Can you work these out from the model? Positions are in its coordinate system, mm. Face numbers are marked on the shaded views. A direction names the side the tool comes from. Round coordinates to 2 decimals unless told otherwise and drop trailing zeros. Order: outer loops, then holes, each group sorted by start corner. A loop starts at its lowest first (then second) coordinate and runs counter-clockwise, first axis right, second up. Notation, with made-up numbers: (6.25, 24.5) -> (43.25, 24.5) arc R19 ccw to (43.25, 30.5) -> close; hole circle Ø2 at (57, 17). An arc over 180 degrees is marked (long way). Use a Markdown table: item, result. Add a question column.
Q1. If we section it at A-A on x = 3.5: List the corners of the cut face in (y, z) for me.
Q2. I need wall thicknesses on line 1 along Z through (x, y) = (-6.5, 7.25); line 2 along Z through (x, y) = (-3, 15); line 3 along X through (y, z) = (7.25, 32). Which ranges of each line are inside material? Lowest first, please. Write a range as [from, to].
Q3. I'm going to push flat-ended pins straight in: pin 1 Ø2 at (y, z) = (14.5, 20.5) entering from +X; pin 2 Ø4 at (y, z) = (7.5, 8.5) entering from -X; pin 3 Ø1 at (x, y) = (-12, 7.5) entering from -Z. Where does each tip first touch, or does it pass through?
Q4. If we section it at C-C on z = 52.5: List the corners of the cut face in (x, y) for me.
Q5. If we section it at D-D on y = 3: List the corners of the cut face in (x, z) for me.
Q6. If we section it at B-B on y = 8.75: List the corners of the cut face in (x, z) for me.
Q7. We'd pull the mould along X, two halves only. Please class the marked faces 1, 2 and 3: +X half, -X half, draft (parallel to the pull), parting line (faces both ways), or undercut.
Q8. For the marked faces 4, 5 and 6, which set-ups out of +Z, -Z, +X, -X, +Y, -Y let a thin tool reach every point of the face, with its end or its side?
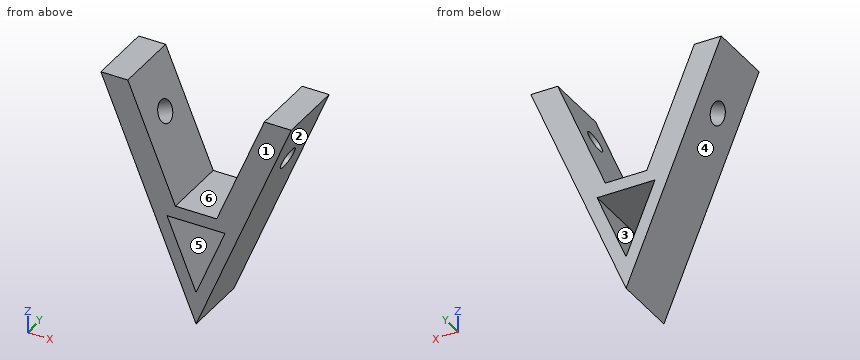
```python
from build123d import *

# Parameters (mm, degrees)
BOSS_EXTRUDE1_DEPTH = 16
CUT_EXTRUDE1_DEPTH  = 16
SKETCH3_R           = 2.65
CUT_EXTRUDE2_DEPTH  = 16
SKETCH4_R           = 2.65
CUT_EXTRUDE3_DEPTH  = 16


with BuildPart() as part:
    # Sketch1 → Boss-Extrude1 (new body)
    with BuildSketch(Plane(origin=(0, 0, 0), x_dir=(1, 0, 0), z_dir=(0, 1, 0))):
        Polygon((0, 0), (-22.961005942, -55.432771951), (22.961005942, -55.432771951), align=None)
    extrude(amount=BOSS_EXTRUDE1_DEPTH)

    # Sketch2 → Cut-Extrude1 (cut)
    with BuildSketch(Plane(origin=(0, 16, 0), x_dir=(1, 0, 0), z_dir=(0, 1, 0))):
        Polygon((-16.46665274, -55.432771951), (-4.986149769, -27.716385975), (4.986149769, -27.716385975), (16.46665274, -55.432771951), align=None)
        Polygon((-6.990685683, -24.716385975), (6.990685683, -24.716385975), (0, -7.839377789), align=None)
    extrude(amount=-CUT_EXTRUDE1_DEPTH, mode=Mode.SUBTRACT)

    # Sketch3 → Cut-Extrude2 (cut)
    with BuildSketch(Plane(origin=(0, 0, 0), x_dir=(-0.3826834323650873, 0, -0.9238795325112878), z_dir=(0.9238795325112878, 0, -0.3826834323650873))):
        with Locations((-45.85, 8)):
            Circle(SKETCH3_R)
    extrude(amount=-CUT_EXTRUDE2_DEPTH, mode=Mode.SUBTRACT)

    # Sketch4 → Cut-Extrude3 (cut)
    with BuildSketch(Plane(origin=(0, 0, 0), x_dir=(-0.3826834323650873, 0, 0.9238795325112878), z_dir=(-0.9238795325112878, 0, -0.3826834323650873))):
        with Locations((45.85, 8)):
            Circle(SKETCH4_R)
    extrude(amount=-CUT_EXTRUDE3_DEPTH, mode=Mode.SUBTRACT)


solid = part.part
```
Answer below:
| question | item | result |
|---|---|---|
| 1 | outline | (0, 8.45) -> (16, 8.45) -> (16, 16.29) -> (0, 16.29) -> close; (0, 24.72) -> (16, 24.72) -> (16, 27.72) -> (0, 27.72) -> close |
| 2 | line 1 | [15.69, 23.53], [24.72, 31.37] |
| 2 | line 2 | [7.24, 15.08], [24.72, 27.72] |
| 2 | line 3 | [-13.25, -6.76], [6.76, 13.25] |
| 3 | pin 1 | x = 8.91 |
| 3 | pin 2 | x = -4.35 |
| 3 | pin 3 | z = 27.76 |
| 4 | outline | (-21.75, 0) -> (-15.25, 0) -> (-15.25, 16) -> (-21.75, 16) -> close; (15.25, 0) -> (21.75, 0) -> (21.75, 16) -> (15.25, 16) -> close |
| 5 | outline | (-22.96, 55.43) -> (0, 0) -> (22.96, 55.43) -> (16.47, 55.43) -> (4.99, 27.72) -> (-4.99, 27.72) -> (-16.47, 55.43) -> close; hole (-6.99, 24.72) -> (0, 7.84) -> (6.99, 24.72) -> close |
| 6 | outline | (-22.96, 55.43) -> (-18.52, 44.71) -> (-12.98, 47) -> (-16.47, 55.43) -> close; (-16.57, 40.01) -> (0, 0) -> (16.57, 40.01) -> (11.03, 42.31) -> (4.99, 27.72) -> (-4.99, 27.72) -> (-11.03, 42.31) -> close; (12.98, 47) -> (18.52, 44.71) -> (22.96, 55.43) -> (16.47, 55.43) -> close; hole (-6.99, 24.72) -> (0, 7.84) -> (6.99, 24.72) -> close |
| 7 | face 1 | draft |
| 7 | face 2 | +X half |
| 7 | face 3 | undercut |
| 8 | face 4 | -Z, -X, +Y, -Y |
| 8 | face 5 | +Y, -Y |
| 8 | face 6 | +Z, +Y, -Y |
